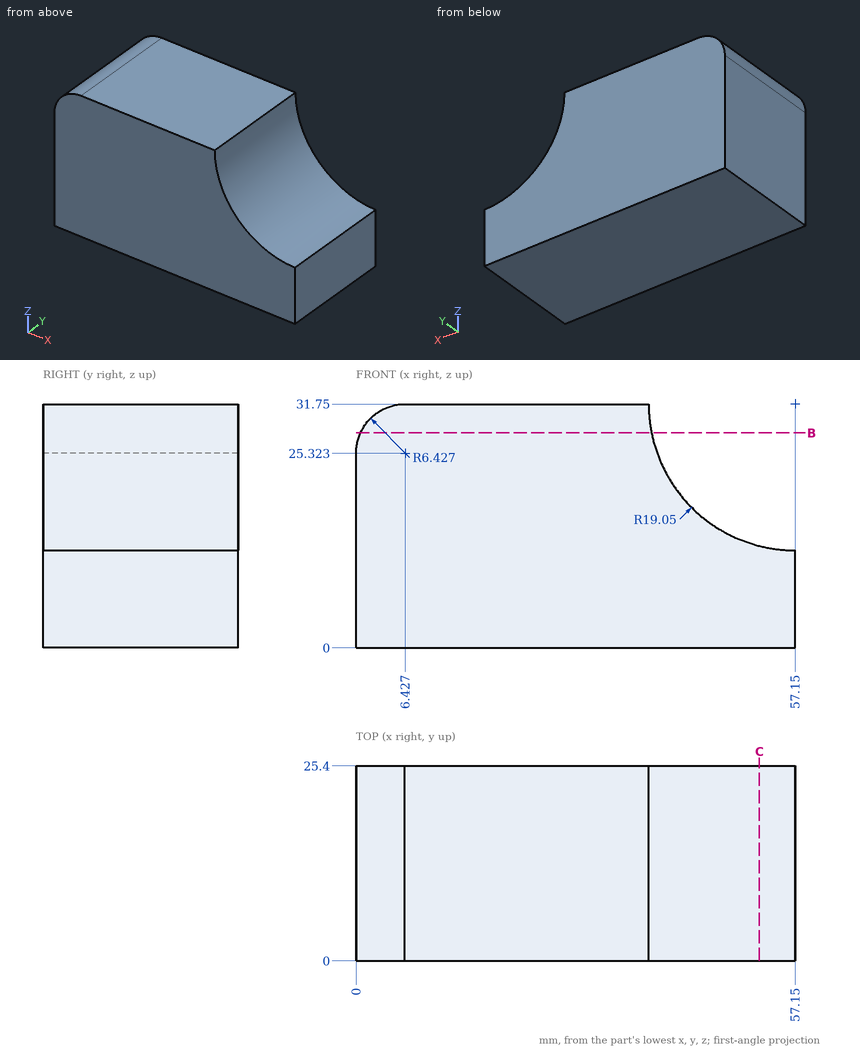
The drawing under review shows one solid part. Ordinate dimensions are in mm from its lowest x, y, z. Coordinates: 2 decimals unless noted, no trailing zeros. Order: outer loops, then holes, each group sorted by start corner. A loop starts at its lowest first (then second) coordinate and runs counter-clockwise, first axis right, second up. Notation, with made-up numbers: M -5.75,41 L 25.25,41 A20 cw 25.25,76 Z; hole C 46.25,6 d11. An arc over 180 degrees is marked long. One line per question, with ' | ' between items.
(1) For probe 1 along X at (y, z) = (20.5, 30); probe 2 along X at (y, z) = (5.25, 27); probe 3 along Z at (x, y) = (46, 18.5) (1 decimal), list the stretches that pass through material, from the lowest coordinate up. Write a range as from..to.
Geometry results:
probe 1: x = 2.02..38.18 | probe 2: x = 0.22..38.7 | probe 3: z = 0..16.3
(2) Add section C-C, the plane x = 52.5. Write out the cut boundary in (y, z).
Geometry results:
outline: M 0,0 L 25.4,0 L 25.4,13.28 L 0,13.28 Z
(3) Insertion check: pin 1 (4 mm diameter, centred on x = 48.5, y = 4, fed in from +Z) (1 decimal); pin 2 (2 mm diameter, centred on y = 11, z = 26, fed in from +X). Each pin has a flat end and moves straight along its axis. Give the tip position at first contact, or say it passes through.
Geometry results:
pin 1: stops at z = 16 | pin 2: stops at x = 39.34
(4) Add section B-B, the plane z = 28. Write out the cut boundary in (x, y), then the cut area to 3 significant figures.
Geometry results:
outline: M 0.58,0 L 38.47,0 L 38.47,25.4 L 0.58,25.4 Z | area: 962 mm²
